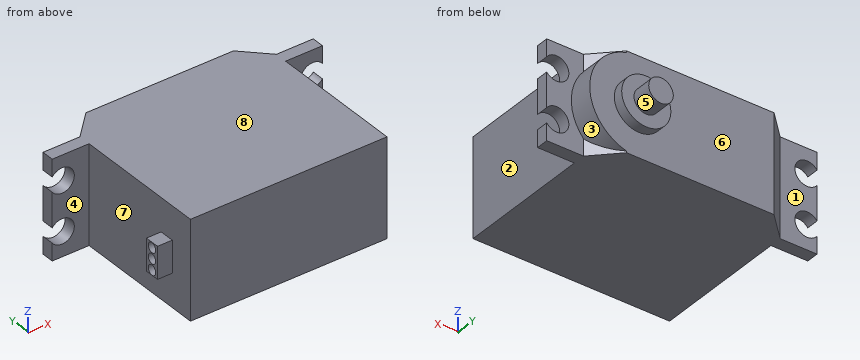
Autodesk Inventor part; units mm, degrees
ref_plane "YZ Plane" through (0, 0, 0) normal (1, 0, 0) x (0, 1, 0)
ref_plane "XZ Plane" through (0, 0, 0) normal (0, 1, 0) x (-1, 0, 0)
ref_plane "XY Plane" through (0, 0, 0) normal (0, 0, 1) x (1, 0, 0)
sketch "Sketch1" plane through (0, 0, 0) normal (0, 1, 0) x (-1, 0, 0)
  line L0 (20, -10) -> (-20, -10)
  line L1 (-20, -10) -> (-20, 10)
  line L2 (-20, 10) -> (20, 10)
  line L3 (20, 10) -> (20, -10)
  line L4 (20, -10) -> (-20, 10) construction
  line L5 (-20, -10) -> (20, 10) construction
  point P0 (0, 0)
  dimension "d0" = 40
  dimension "d1" = 20
extrude "Extrusion1" add sketch "Sketch1" along normal blind 30
sketch "Sketch2" plane through (20, 0, 10) normal (1, 0, 0) x (0, 0, -1)
  line L0 (0, 0) -> (0, 30)
  line L1 (20, 30) -> (0, 30)
  line L2 (0, 30) -> (0, 27.5)
  line L3 (0, 27.5) -> (20, 27.5)
  line L4 (20, 27.5) -> (20, 30)
  point P0 (10, 0)
  dimension "d4" = 2.5
extrude "Extrusion2" add sketch "Sketch2" along normal blind 7.5
sketch "Sketch3" plane through (-20, 0, -10) normal (-1, 0, 0) x (0, 0, 1)
  line L0 (20, 0) -> (20, 30)
  line L1 (0, 30) -> (20, 30)
  line L2 (20, 30) -> (20, 27.5)
  line L3 (20, 27.5) -> (0, 27.5)
  line L4 (0, 27.5) -> (0, 30)
  point P0 (10, 0)
  dimension "d7" = 2.5
extrude "Extrusion3" add sketch "Sketch3" along normal blind 7.5
sketch "Sketch4" plane through (0, 30, 0) normal (0, 1, 0) x (1, 0, 0)
  line L0 (20, 10) -> (-20, 10)
  line L1 (-20, 10) -> (-20, -10)
  line L2 (-20, -10) -> (20, -10)
  line L3 (20, -10) -> (20, 10)
  line L4 (20, 10) -> (-20, -10) construction
  line L5 (-20, 10) -> (20, -10) construction
  point P0 (0, 0)
extrude "Extrusion4" add sketch "Sketch4" along normal blind 5
chamfer "Chamfer1" distance 5 angle 45 1 edges at (-20, 35, 0)
chamfer "Chamfer2" distance 5 angle 45 1 edges at (20, 35, 0)
sketch "Sketch5" plane through (0, 35, 0) normal (0, 1, 0) x (1, 0, 0)
  circle A0 centre (12.5, 0) radius 10
  line L0 (15, 10) -> (-15, 10)
  line L1 (27.5, 10) -> (27.5, -10)
  point P0 (0, 0)
  dimension "d18" = 15
extrude "Extrusion5" add sketch "Sketch5" against normal blind 5
sketch "Sketch6" plane through (0, 30, 0) normal (0, 1, 0) x (1, 0, 0)
  circle A0 centre (25.5, -5) radius 2.5
  line L0 (27.5, -10) -> (20, -10)
  line L1 (27.5, -10) -> (27.5, 10)
  circle A1 centre (25.5, 5) radius 2.5
  line L2 (20, 10) -> (27.5, 10)
  point P0 (0, 0)
  dimension "d21" = 5
  dimension "d22" = 5
  dimension "d23" = 2
  dimension "d24" = 5
  dimension "d25" = 5
  dimension "d26" = 2
extrude "Extrusion6" cut sketch "Sketch6" against normal blind 5
sketch "Sketch7" plane through (0, 30, 0) normal (0, 1, 0) x (1, 0, 0)
  circle A0 centre (-25.5, 5) radius 2.5
  circle A1 centre (-25.5, -5) radius 2.5
  line L0 (-27.5, -10) -> (-27.5, 10)
  line L1 (-20, -10) -> (-27.5, -10)
  line L2 (-27.5, 10) -> (-20, 10)
  point P0 (0, 0)
  dimension "d29" = 5
  dimension "d30" = 5
  dimension "d31" = 2
  dimension "d32" = 2
  dimension "d33" = 5
  dimension "d34" = 5
extrude "Extrusion7" cut sketch "Sketch7" against normal blind 5
sketch "Sketch8" plane through (0, 35, 0) normal (0, 1, 0) x (1, 0, 0)
  circle A0 centre (12.5, 0) radius 5
  line L0 (27.5, 3.5) -> (27.5, -3.5)
  point P0 (0, 0)
  dimension "d37" = 10
  dimension "d38" = 15
extrude "Extrusion8" add sketch "Sketch8" along normal blind 2
sketch "Sketch9" plane through (12.5, 37, 0) normal (0, 1, 0) x (1, 0, 0)
  circle A0 centre (0, 0) radius 2.5
  point P0 (-12.5, 0)
  dimension "d41" = 5
extrude "Extrusion9" add sketch "Sketch9" along normal blind 4
sketch "Sketch10" plane through (-20, 0, -10) normal (-1, 0, 0) x (0, 0, 1)
  line L0 (13.25, 7.9352) -> (6.75, 7.9352)
  line L1 (6.75, 7.9352) -> (6.75, 4.9352)
  line L2 (6.75, 4.9352) -> (13.25, 4.9352)
  line L3 (13.25, 4.9352) -> (13.25, 7.9352)
  line L4 (13.25, 7.9352) -> (6.75, 4.9352) construction
  line L5 (6.75, 7.9352) -> (13.25, 4.9352) construction
  circle A0 centre (10, 6.4352) radius 1
  circle A1 centre (12.1728, 6.4352) radius 1
  circle A2 centre (7.7773, 6.4352) radius 1
  point P0 (10, 0)
  dimension "d44" = 6.5
  dimension "d45" = 3
  dimension "d46" = 2
  dimension "d47" = 2
  dimension "d48" = 2
extrude "Extrusion10" add sketch "Sketch10" along normal blind 3
sketch "Sketch11" plane through (0, 30, 0) normal (0, 1, 0) x (1, 0, 0)
  point P0 (0, 0)
properties part number "block"
Input: part model. Units: mm. Frame: model coordinates. Face numbers are marked on the shaded views. A direction names the side the tool comes from. Coordinates: 2 decimals unless noted, no trailing zeros. Loops run counter-clockwise (first coordinate to the right, second up) from the corner with the lowest first, then second, coordinate; pieces in that order, holes last. Notation, with made-up numbers: (19, -4.75) - (43, -4.75) arc R31 ccw to (43, 28.25) - close; hole circle Ø6 at (27.25, -17.5). An arc over 180 degrees is marked (long way). Answer in a Markdown table with one row per item.
(1) Cut plane D-D on y = 23. Output: boundary loops of the cut face in (x, z), plus the area to 3 significant figures.
Model answer:
| item | result |
|---|---|
| outline | (-20, -10) - (20, -10) - (20, 10) - (-20, 10) - close |
| area | 800 mm² |
(2) Set-up query: the marked faces 1, 2, 3, 4 and 5. Return all of +Z, -Z, +X, -X, +Y, -Y with unobstructed straight access to the full face (end or side cutting, diameter ignored); none if empty.
Model answer:
| item | result |
|---|---|
| face 1 | +Z, -Z, -X, +Y |
| face 2 | +Z, -Z, +X, -Y |
| face 3 | +X, +Y |
| face 4 | +Z, -Z, -X |
| face 5 | +Y |
(3) Material intervals for L1, parallel to Z at x = 25.5, y = 28.65; L2, parallel to Z at x = -25, y = 28; L3, parallel to X at y = 17.5, z = -8, sorted ascending. Write a range as from..to.
Model answer:
| item | result |
|---|---|
| L1 | z = -10..-7.5, -2.5..2.5, 7.5..10 |
| L2 | z = -10..-7.45, -2.55..2.55, 7.45..10 |
| L3 | x = -20..20 |
(4) Cut plane C-C on x = 12.5. Output: boundary loops of the cut face in (y, z), plus the area to 3 significant figures.
Model answer:
| item | result |
|---|---|
| outline | (0, -10) - (35, -10) - (35, -5) - (37, -5) - (37, -2.5) - (41, -2.5) - (41, 2.5) - (37, 2.5) - (37, 5) - (35, 5) - (35, 10) - (0, 10) - close |
| area | 740 mm² |
(5) Pin query (flat end, axial travel): P1, Ø2, axis at x = -23.5, z = -4.5, coming from the +Y side; P2, Ø12, axis at y = 35, z = 3, coming from the -X side; P3, Ø3.5, axis at x = -22, z = 0.5, coming from the -Y side; P4, Ø1.2, axis at y = 6.44, z = 0, coming from the +X side. Return the tip coordinate at first contact, or that it passes through.
Model answer:
| item | result |
|---|---|
| P1 | stops at y = 30 |
| P2 | stops at x = -27.5 |
| P3 | stops at y = 4.94 |
| P4 | stops at x = 20 |
(6) Cut plane A-A on x = 25.5. Output: boundary loops of the cut face in (y, z).
Model answer:
| item | result |
|---|---|
| outline | (27.5, -10) - (30, -10) - (30, -7.5) - (27.5, -7.5) - close; (27.5, -2.5) - (30, -2.5) - (30, 2.5) - (27.5, 2.5) - close; (27.5, 7.5) - (30, 7.5) - (30, 10) - (27.5, 10) - close |
(7) Mould query, pull axis Y, two halves, no side actions, for the marked faces 6, 7 and 8. Classes: pulls with the +Y half, pulls with the -Y half, needs draft (parallel to the pull), parting line crosses it, or undercut.
Model answer:
| item | result |
|---|---|
| face 6 | pulls with the +Y half |
| face 7 | undercut |
| face 8 | needs draft |
